Check sheet for the modelled part. Datum: model origin and axes. Units: mm. A direction names the side the tool comes from. Give positions to 0.01 mm unless a question says otherwise; leave off trailing zeros. Loops run counter-clockwise (first coordinate to the right, second up) from the corner with the lowest first, then second, coordinate; pieces in that order, holes last. Notation, with made-up numbers: M 25.5,38.5 L 72.5,38.5 A17 ccw 72.5,43.5 Z; hole C 68.5,53 d6. An arc over 180 degrees is marked long. Use one line per item in the form item = value.
from build123d import *

# Parameters (mm, degrees)
SKETCH1_W           = 63.5
SKETCH1_H           = 63.5
SKETCH1_W_2         = 50.8
SKETCH1_H_2         = 50.8
BOSS_EXTRUDE1_DEPTH = 50.8
SKETCH2_W           = 63.5
SKETCH2_H           = 63.5
BOSS_EXTRUDE3_DEPTH = 6.35
SKETCH3_W           = 63.5
SKETCH3_H           = 63.5
BOSS_EXTRUDE4_DEPTH = 52.3494
SKETCH4_R           = 22.9997
CUT_EXTRUDE1_DEPTH  = 139.883012281
FILLET2_R           = 31.75
SKETCH5_W           = 12.7
SKETCH5_H           = 12.7
BOSS_EXTRUDE5_DEPTH = 25.4
FILLET3_R           = 12.7


with BuildPart() as part:
    # Sketch1 → Boss-Extrude1 (new body)
    with BuildSketch(Plane(origin=(0, 0, 0), x_dir=(1, 0, 0), z_dir=(0, 1, 0))):
        with Locations((25.4, 25.4)):
            Rectangle(SKETCH1_W, SKETCH1_H)
        with Locations((25.4, 25.4)):
            Rectangle(SKETCH1_W_2, SKETCH1_H_2, mode=Mode.SUBTRACT)
    extrude(amount=BOSS_EXTRUDE1_DEPTH)

    # Sketch2 → Boss-Extrude3 (add)
    with BuildSketch(Plane(origin=(0, 50.8, 0), x_dir=(1, 0, 0), z_dir=(0, 1, 0))):
        with Locations((25.4, 25.4)):
            Rectangle(SKETCH2_W, SKETCH2_H)
    extrude(amount=BOSS_EXTRUDE3_DEPTH)

    # Sketch3 → Boss-Extrude4 (add)
    with BuildSketch(Plane(origin=(0, 57.15, 0), x_dir=(1, 0, 0), z_dir=(0, 1, 0))):
        with Locations((25.4, 25.4)):
            Rectangle(SKETCH3_W, SKETCH3_H)
    extrude(amount=BOSS_EXTRUDE4_DEPTH)

    # Sketch4 → Cut-Extrude1 (cut, through all)
    with BuildSketch(Plane.XY.offset(6.35)):
        with Locations((25.4, 80.1497)):
            Circle(SKETCH4_R)
    extrude(amount=-CUT_EXTRUDE1_DEPTH, mode=Mode.SUBTRACT)

    # Fillet2
    fillet2_edges = [part.edges().sort_by_distance(p)[0] for p in [
        (-6.35, 109.4994, -25.4),
        (57.15, 109.4994, -25.4),
    ]]
    fillet(fillet2_edges, radius=FILLET2_R - 0.0001)  # a hair under: the kernel refuses the full size

    # Sketch5 → Boss-Extrude5 (add)
    with BuildSketch(Plane.XY.offset(6.35)):
        with Locations((0, 6.35)):
            Rectangle(SKETCH5_W, SKETCH5_H)
    extrude(amount=BOSS_EXTRUDE5_DEPTH)

    # Fillet3
    fillet3_edges = [part.edges().sort_by_distance(p)[0] for p in [
        (6.35, 6.35, 6.35),
        (0, 12.7, 6.35),
    ]]
    fillet(fillet3_edges, radius=FILLET3_R)


solid = part.part
1) Depth check by flat-ended pin: pin 1 Ø8 at (x, y) = (30, 30) entering from +Z; pin 2 Ø14 at (y, z) = (7, 25.5) entering from +X; pin 3 Ø1.5 at (x, z) = (38, -3.5) entering from -Y; pin 4 Ø19 at (x, y) = (21.5, 71.5) entering from +Z. Enter the tip coordinate at first touch or a pass-through.
Evaluation:
pin_1 = 6.35
pin_2 = 6.36
pin_3 = 50.8
pin_4 = through
2) Release check for a two-part mould opening along X. For faces 5 (the face through (18.2, 0, 0.3)), 6 (the face through (37.765, 99.543, -24.956)), 7 (the face through (47.6, 100.45, -25.84)) record: pulls with the +X half, pulls with the -X half, needs draft (parallel to the pull), parting line crosses it, or undercut.
Evaluation:
face_5 = needs draft
face_6 = undercut
face_7 = pulls with the +X half
3) Section check B-B (x = 8). Record the cut outline in (y, z).
Evaluation:
outline = M 0,-57.15 L 65.11,-57.15 L 65.11,6.35 L 25.4,6.35 A12.7 cw 14.35,12.79 L 0,12.79 L 0,0 L 50.8,0 L 50.8,-50.8 L 0,-50.8 Z; M 95.19,-57.15 L 104.31,-57.15 L 104.31,6.35 L 95.19,6.35 Z
4) Section check C-C (y = 69). Record the cut outline in (x, z).
Evaluation:
outline = M -6.35,-57.15 L 5.28,-57.15 L 5.28,6.35 L -6.35,6.35 Z; M 45.52,-57.15 L 57.15,-57.15 L 57.15,6.35 L 45.52,6.35 Z
5) Section check A-A (y = 34.5). Record the cut outline in (x, z), then the cut area to 3 significant figures.
Evaluation:
outline = M -6.35,-57.15 L 57.15,-57.15 L 57.15,6.35 L -6.35,6.35 Z; hole M 0,-50.8 L 50.8,-50.8 L 50.8,0 L 0,0 Z
area = 1,450 mm^2
6) Scan lines: line 1 (Y direction, x = 25.4, z = -9); line 2 (Z direction, x = 11, y = 48); line 3 (X direction, y = 16, z = -36.5). Record each from-to range of solid material in increasing order.
Evaluation:
line_1 = 50.8 to 57.15, 103.15 to 109.5
line_2 = -57.15 to -50.8, 0 to 6.35
line_3 = -6.35 to 0, 50.8 to 57.15
7) Set-up check for faces 1 (the face through (0, 12.7, 25)), 2 (the face through (25, 25, -50.8)), 3 (the face through (6.35, 6, 25)), 4 (the face through (25, 42, 6.35)): record each of +Z, -Z, +X, -X, +Y, -Y from which the full face is reachable in a straight line by a thin tool's end or side.
Evaluation:
face_1 = +Z, +X, -X, +Y
face_2 = -Y
face_3 = +Z, +X, +Y, -Y
face_4 = +Z, +X, +Y
